Can you work these out from the drawing? Everything is in mm from the part's minimum corner. A direction names the side the tool comes from. Round coordinates to 2 decimals unless told otherwise and drop trailing zeros. Loops run counter-clockwise (first coordinate to the right, second up) from the corner with the lowest first, then second, coordinate; pieces in that order, holes last. Notation, with made-up numbers: (47.25, 58.25) -> (83.25, 58.25) arc R7 cw to (83.25, 65.25) -> close; hole circle Ø7 at (66, 13). An arc over 180 degrees is marked (long way). One line per item, written item: value.
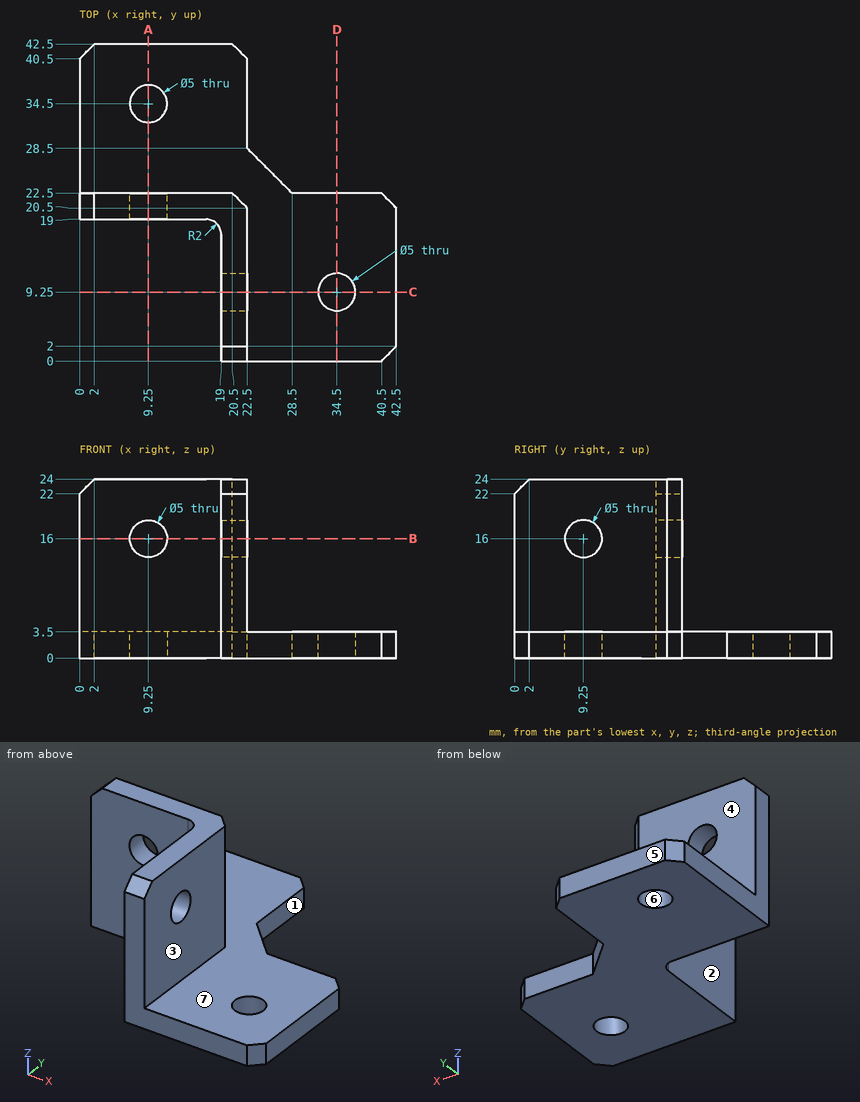
Item 1: For the marked faces 1, 2, 3 and 4, which set-ups out of +Z, -Z, +X, -X, +Y, -Y let a thin tool reach every point of the face, with its end or its side?
Output:
face 1: +Z, -Z, +X, +Y
face 2: +Z, -Z, -X, -Y
face 3: +Z, +X, +Y, -Y
face 4: +Z, +X, -X, +Y
Item 2: Will these pins go through, and if not, where does the flat tip stop? pin 1 Ø5 at (y, z) = (7.5, 13) entering from -X; pin 2 Ø4 at (x, z) = (19.5, 7) entering from +Y; pin 3 Ø6 at (x, z) = (9.25, 16) entering from -Y.
Output:
pin 1: stops at x = 19
pin 2: stops at y = 22.5
pin 3: stops at y = 19
Item 3: If we section it at A-A on x = 9.25: List the corners of the cut face in (y, z) for me.
Output:
outline: (19, 0) -> (32, 0) -> (32, 3.5) -> (22.5, 3.5) -> (22.5, 13.5) -> (19, 13.5) -> close; (19, 18.5) -> (22.5, 18.5) -> (22.5, 24) -> (19, 24) -> close; (37, 0) -> (42.5, 0) -> (42.5, 3.5) -> (37, 3.5) -> close
Item 4: If we mould it in two halves opening along Y, with no side actions, what happens to the marked faces 5, 6 and 7? For each: released by +Y, released by -Y, zero draft, split by the parting line, or undercut.
Output:
face 5: released by +Y
face 6: undercut
face 7: zero draft
Item 5: If we section it at D-D on x = 34.5: List the corners of the cut face in (y, z) for me.
Output:
outline: (0, 0) -> (6.75, 0) -> (6.75, 3.5) -> (0, 3.5) -> close; (11.75, 0) -> (22.5, 0) -> (22.5, 3.5) -> (11.75, 3.5) -> close
Item 6: If we section it at B-B on z = 16: List the corners of the cut face in (x, y) for me.
Output:
outline: (0, 19) -> (6.75, 19) -> (6.75, 22.5) -> (0, 22.5) -> close; (11.75, 19) -> (17, 19) arc R2 cw to (19, 17) -> (19, 11.75) -> (22.5, 11.75) -> (22.5, 20.5) -> (20.5, 22.5) -> (11.75, 22.5) -> close; (19, 0) -> (22.5, 0) -> (22.5, 6.75) -> (19, 6.75) -> close
Item 7: I need wall thicknesses on line 1 (Y direction, x = 19.5, z = 15.75); line 2 (Z direction, x = 9, y = 21); line 3 (Y direction, x = 9.25, z = 1.85). Which ranges of each line are inside material? Lowest first, please. Write a range as from..to.
Output:
line 1: y = 0..6.76, 11.74..22.5
line 2: z = 0..13.51, 18.49..24
line 3: y = 19..32, 37..42.5
